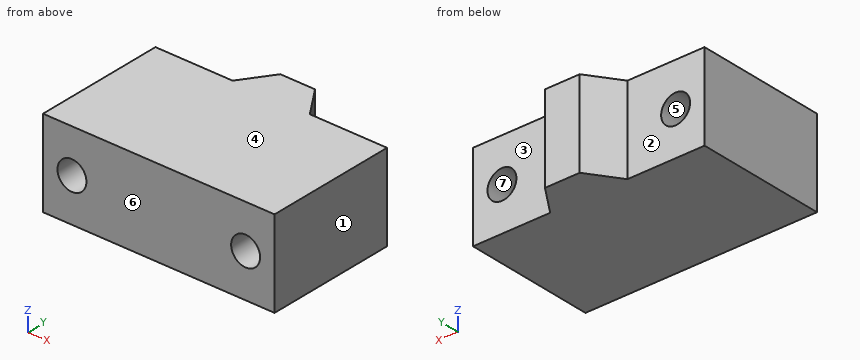
from build123d import *

# Parameters (mm, degrees)
BOSS_EXTRU_1_DEPTH      = 45
ESQUISSE2_R             = 7.5
BOSS_EXTRU_2_DEPTH      = 68
ESQUISSE2_4_R           = 7.5
ENL_V_MAT_EXTRU_1_DEPTH = 69


with BuildPart() as part:
    # Esquisse1 → Boss.-Extru.1 (new body)
    with BuildSketch(Plane.XY):
        Polygon((0, 0), (120, 0), (120, 68), (80, 68), (69, 84), (51, 84), (40, 68), (0, 68), align=None)
    extrude(amount=BOSS_EXTRU_1_DEPTH)

    # Esquisse2 → Boss.-Extru.2 (add, through all)
    with BuildSketch(Plane(origin=(0, 68, 0), x_dir=(1, 0, 0), z_dir=(0, 1, 0))):
        with Locations((105, -22.5)):
            Circle(ESQUISSE2_R)
        with Locations((15, -22.5)):
            Circle(ESQUISSE2_R)
    extrude(amount=-BOSS_EXTRU_2_DEPTH)

    # Esquisse2_4 → Enl_v. mat.-Extru.1 (cut, through all)
    with BuildSketch(Plane(origin=(0, 68, 0), x_dir=(1, 0, 0), z_dir=(0, 1, 0))):
        with Locations(Location((105, -22.5, 0), (0, 0, 180))):  # turned: the seam where the file's is
            Circle(ESQUISSE2_4_R)
        with Locations(Location((15, -22.5, 0), (0, 0, 180))):  # turned: the seam where the file's is
            Circle(ESQUISSE2_4_R)
    extrude(amount=-ENL_V_MAT_EXTRU_1_DEPTH, mode=Mode.SUBTRACT)


solid = part.part
The model under review builds one solid part; all positions refer to its coordinate system, in mm. Face numbers are marked on the shaded views. A direction names the side the tool comes from. Round coordinates to 2 decimals unless told otherwise and drop trailing zeros. Write each loop counter-clockwise with the first axis right and the second up, starting at its lowest first coordinate (ties: lowest second). Pieces come first, ordered by that corner, then holes. Notation, with made-up numbers: (39, 72.25) - (97, 72.25) arc R31 cw to (97, 96.25) - close; hole circle Ø6 at (-20.75, 77.25). An arc over 180 degrees is marked (long way). One line per item, written item: value. Start each with the question number.
1. Consider section D-D on z = 35. Write out the cut boundary in (x, y).
2. Clearance check with flat-ended pins moving along their axes: P1, Ø20, axis at x = 18, z = 26, coming from the +Y side; P2, Ø6, axis at x = 73.5, z = 21, coming from the +Y side; P3, Ø13.5, axis at x = 105, z = 22.5, coming from the +Y side. State where each tip first meets the part, or that it passes through.
3. The part is to be moulded in two halves that separate along Z. For the marked faces 4, 5, 6 and 7, say which applies: released by +Z, released by -Z, zero draft, split by the parting line, or undercut.
4. To check wall thickness, follow L1, parallel to X at y = 38, z = 22; L2, parallel to X at y = 59, z = 18.5; L3, parallel to Z at x = 15, y = 50. State the ranges of each line that lie inside material, in increasing order. Write a range as from..to.
5. Consider section A-A on z = 22.5. Write out the cut boundary in (x, y).
6. Machinability: for the marked faces 1, 2 and 3, which of the approach directions +Z, -Z, +X, -X, +Y, -Y give a long, thin tool a straight path to every point of the face, cutting with its end or side? Answer none if there is none.
7. Consider section C-C on x = 15. Write out the cut boundary in (y, z).
8. Consider section B-B on y = 61. Write out the cut boundary in (x, z), and give its area (3 significant figures).
Checks:
1. outline: (0, 0) - (120, 0) - (120, 68) - (80, 68) - (69, 84) - (51, 84) - (40, 68) - (0, 68) - close
2. P1: stops at y = 68
2. P2: stops at y = 81.82
2. P3: passes through
3. face 4: released by +Z
3. face 5: undercut
3. face 6: zero draft
3. face 7: undercut
4. L1: x = 0..7.52, 22.48..97.52, 112.48..120
4. L2: x = 0..8.66, 21.34..98.66, 111.34..120
4. L3: z = 0..15, 30..45
5. outline: (0, 0) - (7.5, 0) - (7.5, 68) - (0, 68) - close; (22.5, 0) - (97.5, 0) - (97.5, 68) - (80, 68) - (69, 84) - (51, 84) - (40, 68) - (22.5, 68) - close; (112.5, 0) - (120, 0) - (120, 68) - (112.5, 68) - close
6. face 1: +Z, -Z, +X, +Y, -Y
6. face 2: +Z, -Z, -X, +Y
6. face 3: +Z, -Z, +X, +Y
7. outline: (0, 0) - (68, 0) - (68, 15) - (0, 15) - close; (0, 30) - (68, 30) - (68, 45) - (0, 45) - close
8. outline: (0, 0) - (120, 0) - (120, 45) - (0, 45) - close; hole circle Ø15 at (15, 22.5); hole circle Ø15 at (105, 22.5)
8. area: 5,050 mm^2
